Autodesk Inventor part; units mm, degrees
ref_plane "YZ Plane" through (0, 0, 0) normal (1, 0, 0) x (0, 1, 0)
ref_plane "XZ Plane" through (0, 0, 0) normal (0, 1, 0) x (-1, 0, 0)
ref_plane "XY Plane" through (0, 0, 0) normal (0, 0, 1) x (1, 0, 0)
sketch "Szkic1" plane through (0, 0, 0) normal (0, 0, 1) x (1, 0, 0)
  line L0 (-211.8041, 0) -> (185.2919, 0) construction
  line L1 (-211.8041, -6.5) -> (185.2919, -6.5)
  line L2 (185.2919, 6.5) -> (-211.8041, 6.5)
  arc A0 (-211.8041, 6.5) -> (-211.8041, -6.5) centre (-211.8041, 0) ccw
  arc A1 (185.2919, -6.5) -> (185.2919, 6.5) centre (185.2919, 0) ccw
  line L3 (-211.8041, 7.9) -> (185.2919, 7.9)
  arc A2 (185.2919, -7.9) -> (185.2919, 7.9) centre (185.2919, 0) ccw
  line L4 (185.2919, -7.9) -> (-211.8041, -7.9)
  arc A3 (-211.8041, 7.9) -> (-211.8041, -7.9) centre (-211.8041, 0) ccw
  point P0 (0, 0)
  point P1 (-13.2561, 0)
  dimension "d0" = 198.548
  dimension "d1" = 13
  dimension "d2" = 1.4
extrude "Wyciągnięcie proste1" add sketch "Szkic1" along normal blind 6.3
properties part number "COTS_GENERIC_X_Axis_Timing_Belt"
Could you check a few things on this model? Use its own coordinates, in mm. A direction names the side the tool comes from. Give positions to 0.01 mm unless a question says otherwise; leave off trailing zeros. Order: outer loops, then holes, each group sorted by start corner. A loop starts at its lowest first (then second) coordinate and runs counter-clockwise, first axis right, second up. Notation, with made-up numbers: (54.5, 0) -> (106.5, 0) arc R25 cw to (106.5, 23) -> close; hole circle Ø11 at (-33, -24). An arc over 180 degrees is marked (long way). Answer in a Markdown table with one row per item. Add a question column.
Item 1: I'm going to push flat-ended pins straight in: P1, Ø1.5, axis at y = -6, z = 1, coming from the -X side; P2, Ø3, axis at y = 4.5, z = 4, coming from the -X side. Where does each tip first touch, or does it pass through?
Item 2: Imagine slicing it at B-B (y = 0). List the corners of the cut face in (x, z) for me, and give its area (3 significant figures).
Item 3: We'd pull the mould along Y, two halves only. Please class faces 1 (the flat face through (-16, 7.9, 3)), 2 (the flat face through (-14, 7, 0)), 3 (the flat face through (-16, -6.5, 3)): pulls with the +Y half, pulls with the -Y half, needs draft (parallel to the pull), parting line crosses it, or undercut.
Item 4: Imagine slicing it at C-C (z = 3.25). List the corners of the cut face in (x, y) for me, and give its area (3 significant figures).
Item 5: Imagine slicing it at A-A (x = 137). List the corners of the cut face in (y, z) for me, and give its area (3 significant figures).
Item 6: For faces 4 (the flat face through (-10, -7.9, 3)), 5 (the cylindrical face through (191.79, 0.14, 3.11)), which set-ups out of +Z, -Z, +X, -X, +Y, -Y let a thin tool reach every point of the face, with its end or its side?
Item 7: Please list where these lines run through material, in increasing order: probe 1 along Y at (x, z) = (81, 4.25); probe 2 along X at (y, z) = (0.5, 2); probe 3 along X at (y, z) = (-0.75, 1.5).
Result:
| question | item | result |
|---|---|---|
| 1 | P1 | x = -217.71 |
| 1 | P2 | x = -219.11 |
| 2 | outline | (-219.7, 0) -> (-218.3, 0) -> (-218.3, 6.3) -> (-219.7, 6.3) -> close; (191.79, 0) -> (193.19, 0) -> (193.19, 6.3) -> (191.79, 6.3) -> close |
| 2 | area | 17.6 mm2 |
| 3 | face 1 | pulls with the +Y half |
| 3 | face 2 | needs draft |
| 3 | face 3 | undercut |
| 4 | outline | (-211.8, -7.9) -> (185.29, -7.9) arc R7.9 ccw to (185.29, 7.9) -> (-211.8, 7.9) arc R7.9 ccw to start; hole (-211.8, -6.5) -> (185.29, -6.5) arc R6.5 ccw to (185.29, 6.5) -> (-211.8, 6.5) arc R6.5 ccw to start |
| 4 | area | 1,180 mm2 |
| 5 | outline | (-7.9, 0) -> (-6.5, 0) -> (-6.5, 6.3) -> (-7.9, 6.3) -> close; (6.5, 0) -> (7.9, 0) -> (7.9, 6.3) -> (6.5, 6.3) -> close |
| 5 | area | 17.6 mm2 |
| 6 | face 4 | +Z, -Z, +X, -X, -Y |
| 6 | face 5 | +Z, -Z |
| 7 | probe 1 | -7.9 to -6.5, 6.5 to 7.9 |
| 7 | probe 2 | -219.69 to -218.28, 191.77 to 193.18 |
| 7 | probe 3 | -219.67 to -218.26, 191.75 to 193.16 |
